CAD build for the part. Positions are in the model's coordinates, mm. Face numbers are marked on the shaded views. A direction names the side the tool comes from. Round coordinates to 2 decimals unless told otherwise and drop trailing zeros. Order: outer loops, then holes, each group sorted by start corner. A loop starts at its lowest first (then second) coordinate and runs counter-clockwise, first axis right, second up. Notation, with made-up numbers: (51.25, -12.5) - (108.25, -12.5) arc R26 cw to (108.25, 2.5) - close; hole circle Ø5 at (58.25, 44). An arc over 180 degrees is marked (long way). Use one line per item in the form item = value. Start each with the question number.
from build123d import *

# Parameters (mm, degrees)
SKETCH_1_R          = 1
EXTRUDE_1_DEPTH     = 6
SKETCH_2_R          = 1.75
EXTRUDE_2_DEPTH     = 0.75
FILLET_1_R          = 0.5
SKETCH_3_W          = 7.004697232
SKETCH_3_H          = 0.75
CUT_EXTRUDE_1_DEPTH = 0.5
SKETCH_4_W          = 0.75
SKETCH_4_H          = 3.75
CUT_EXTRUDE_2_DEPTH = 0.5


with BuildPart() as part:
    # 草图1 → 拉伸1 (new body)
    with BuildSketch(Plane(origin=(0, 0, 0), x_dir=(1, 0, 0), z_dir=(0, 1, 0))):
        with Locations(Location((0, 0, 0), (0, 0, 270))):
            Circle(SKETCH_1_R)
    extrude(amount=EXTRUDE_1_DEPTH)

    # 草图2 → 拉伸2 (add)
    with BuildSketch(Plane(origin=(0, 6, 0), x_dir=(-1, 0, 0), z_dir=(0, 1, 0))):
        with Locations(Location((0, 0, 0), (0, 0, 90))):
            Circle(SKETCH_2_R)
    extrude(amount=EXTRUDE_2_DEPTH)

    # 圆角1
    fillet_1_edges = [part.edges().sort_by_distance(p)[0] for p in [
        (0, 6.75, -1.75),
    ]]
    fillet(fillet_1_edges, radius=FILLET_1_R)

    # 草图3 → 切除-拉伸1 (cut)
    with BuildSketch(Plane(origin=(0, 6.75, 0), x_dir=(-1, 0, 0), z_dir=(0, 1, 0))):
        Rectangle(SKETCH_3_W, SKETCH_3_H)
    extrude(amount=-CUT_EXTRUDE_1_DEPTH, mode=Mode.SUBTRACT)

    # 草图4 → 切除-拉伸2 (cut)
    with BuildSketch(Plane(origin=(0, 6.75, 0), x_dir=(-1, 0, 0), z_dir=(0, 1, 0))):
        Rectangle(SKETCH_4_W, SKETCH_4_H)
    extrude(amount=-CUT_EXTRUDE_2_DEPTH, mode=Mode.SUBTRACT)


solid = part.part
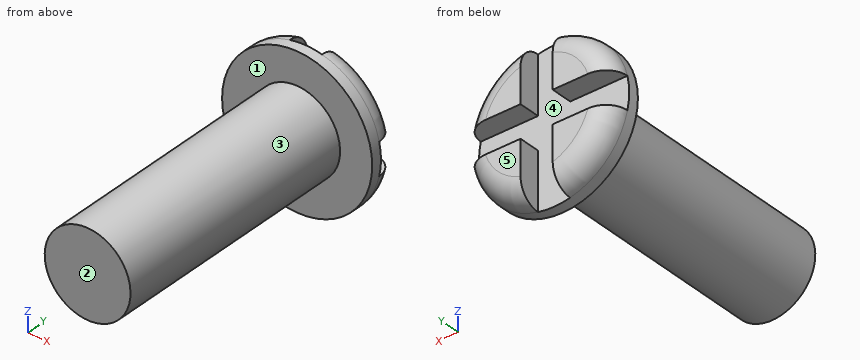
(1) Wall check: line 1 (Y direction, x = -0.05, z = 0.15); line 2 (Y direction, x = 1.1, z = 0.05); line 3 (X direction, y = 5.5, z = 0.85). Give the ranges that are in metal, low to high. Write a range as [from, to].
(2) Slice it at A-A (x = 0). Give the cut face in (y, z).
(3) Slice it at B-B (z = 0). Give the cut face in (x, y).
(4) Slice it at C-C (y = 2.5). Give the cut face in (x, z), and give its area (3 significant figures).
(5) Which spindle directions (+Z, -Z, +X, -X, +Y, -Y) get a long thin tool onto all of the face, cutting with end or side? Do the marked faces 1 and 2. Say none if no direction does.
(6) Mould opens along X. For the marked faces 3, 4 and 5 say: pulls with the +X half, pulls with the -X half, needs draft (parallel to the pull), parting line crosses it, or undercut.
(7) Flat gauge pins, fed straight in: P1, Ø2, axis at x = -1, y = 5.5, coming from the +Z side; P2, Ø0.6, axis at y = 6.5, z = -1, coming from the +X side; P3, Ø0.6, axis at y = 6.5, z = -1, coming from the -X side. Where does each tip first touch, or does it go through?
Results list:
q1.line_1 = [0, 6.25]
q1.line_2 = [6, 6.25]
q1.line_3 = [-0.53, 0.53]
q2.outline = (0, -1) - (6, -1) - (6, -1.75) - (6.25, -1.75) - (6.25, 1.75) - (6, 1.75) - (6, 1) - (0, 1) - close
q3.outline = (-1.75, 6) - (-1, 6) - (-1, 0) - (1, 0) - (1, 6) - (1.75, 6) - (1.75, 6.25) - (-1.75, 6.25) - close
q4.outline = circle Ø2 at (0, 0)
q4.area = 3.14 mm²
q5.face_1 = -Y
q5.face_2 = +Z, -Z, +X, -X, -Y
q6.face_3 = parting line crosses it
q6.face_4 = undercut
q6.face_5 = needs draft
q7.P1 = 1.74
q7.P2 = 1.57
q7.P3 = -1.57
